from build123d import *

# Parameters (mm, degrees)
SKETCH1_R           = 5
BOSS_EXTRUDE1_DEPTH = 100
SKETCH3_R           = 1.1
SKETCH3_R_2         = 0.55
BOSS_EXTRUDE3_DEPTH = 1


with BuildPart() as part:
    # Sketch1 → Boss-Extrude1 (new body)
    with BuildSketch(Plane.XY):
        Circle(SKETCH1_R)
    extrude(amount=BOSS_EXTRUDE1_DEPTH)

    # Sketch3 → Boss-Extrude3 (add)
    with BuildSketch(Plane.XY.offset(100)):
        Circle(SKETCH3_R)
        with Locations((-2.642220318, 1.525486612)):
            Circle(SKETCH3_R_2)
        with Locations((0, 3.050973223)):
            Circle(SKETCH3_R_2)
        with Locations((-2.642220318, -1.525486612)):
            Circle(SKETCH3_R_2)
        with Locations((0, -3.050973223)):
            Circle(SKETCH3_R_2)
        with Locations((2.642220318, -1.525486612)):
            Circle(SKETCH3_R_2)
        with Locations((2.642220318, 1.525486612)):
            Circle(SKETCH3_R_2)
    extrude(amount=BOSS_EXTRUDE3_DEPTH)


solid = part.part
CAD build for the part. Positions are in the model's coordinates, mm. A direction names the side the tool comes from. Give positions to 0.01 mm unless a question says otherwise; leave off trailing zeros. Write each loop counter-clockwise with the first axis right and the second up, starting at its lowest first coordinate (ties: lowest second). Pieces come first, ordered by that corner, then holes. Notation, with made-up numbers: M -22,-38 L 30,-38 A18 ccw 30,-27 Z; hole C 70.25,79.25 d7. An arc over 180 degrees is marked long. Put each result on its own line as item: value. Start each with the question number.
(1) Which spindle directions (+Z, -Z, +X, -X, +Y, -Y) get a long thin tool onto all of the face, cutting with end or side? Do faces 1 (the face through (1, -1, 100)), 2 (the face through (0, 0, 0)). Say none if no direction does.
(2) Flat gauge pins, fed straight in: pin 1 Ø1 at (x, z) = (2.5, 36) entering from +Y; pin 2 Ø1 at (x, z) = (1.5, 47.5) entering from +Y. Where does each tip first touch, or does it go through?
(3) Probe L1, parallel to Z at x = -1.25, y = -3.25; L2, parallel to X at y = 4, z = 7; L3, parallel to X at y = -0.5, z = 18. List the from-to ranges inside material, lowest first.
(4) Band-saw the part on A-A, the plane z = 61. Write the cut outline in (x, y), and give its area (3 significant figures).
Response values:
1. face 1: +Z
1. face 2: -Z, +X, -X, +Y, -Y
2. pin 1: stops at y = 4.58
2. pin 2: stops at y = 4.9
3. L1: z = 0 to 100
3. L2: x = -3 to 3
3. L3: x = -4.97 to 4.97
4. outline: C 0,0 d10
4. area: 78.5 mm2
